Read the model definition and answer for the solid it produces. Units are mm, in the model's axes. Face numbers are marked on the shaded views. A direction names the side the tool comes from. Coordinates: 2 decimals unless noted, no trailing zeros. Order: outer loops, then holes, each group sorted by start corner. A loop starts at its lowest first (then second) coordinate and runs counter-clockwise, first axis right, second up. Notation, with made-up numbers: (77.25, -15) -> (81.25, -15) arc R23 cw to (81.25, 8) -> close; hole circle Ø9 at (78.25, -37). An arc over 180 degrees is marked (long way). Use CSV: the item, a comma, the result in double quotes.
Autodesk Inventor part; units mm, degrees
ref_plane "YZ Plane" through (0, 0, 0) normal (1, 0, 0) x (0, 1, 0)
ref_plane "XZ Plane" through (0, 0, 0) normal (0, 1, 0) x (-1, 0, 0)
ref_plane "XY Plane" through (0, 0, 0) normal (0, 0, 1) x (1, 0, 0)
sketch "Sketch1" plane through (0, 0, 0) normal (0, 0, 1) x (1, 0, 0)
  circle A0 centre (0, 0) radius 16 construction
  line L0 (17.5, 17.5) -> (-17.5, -17.5) construction
  line L1 (-17.5, 17.5) -> (17.5, -17.5) construction
  line L2 (-17, -6) -> (-16.5, -6)
  line L3 (-16, -5.5) -> (-16, 5.5)
  line L4 (-16.5, 6) -> (-17, 6)
  line L5 (-17.5, 12.5) -> (-17.5, 6.5)
  line L6 (-17.5, -6.5) -> (-17.5, -12.5)
  arc A1 (-16.5, -6) -> (-16, -5.5) centre (-16.5, -5.5) ccw
  arc A2 (-16, 5.5) -> (-16.5, 6) centre (-16.5, 5.5) ccw
  arc A3 (-17.5, 6.5) -> (-17, 6) centre (-17, 6.5) ccw
  arc A4 (-17, -6) -> (-17.5, -6.5) centre (-17, -6.5) ccw
  line L7 (6, -17) -> (6, -16.5)
  line L8 (5.5, -16) -> (-5.5, -16)
  line L9 (-6, -16.5) -> (-6, -17)
  arc A5 (6, -16.5) -> (5.5, -16) centre (5.5, -16.5) ccw
  arc A6 (-5.5, -16) -> (-6, -16.5) centre (-5.5, -16.5) ccw
  arc A7 (-6.5, -17.5) -> (-6, -17) centre (-6.5, -17) ccw
  arc A8 (6, -17) -> (6.5, -17.5) centre (6.5, -17) ccw
  line L10 (17, 6) -> (16.5, 6)
  line L11 (16, 5.5) -> (16, -5.5)
  line L12 (16.5, -6) -> (17, -6)
  arc A9 (16.5, 6) -> (16, 5.5) centre (16.5, 5.5) ccw
  arc A10 (16, -5.5) -> (16.5, -6) centre (16.5, -5.5) ccw
  arc A11 (17.5, -6.5) -> (17, -6) centre (17, -6.5) ccw
  arc A12 (17, 6) -> (17.5, 6.5) centre (17, 6.5) ccw
  line L13 (-6, 17) -> (-6, 16.5)
  line L14 (-5.5, 16) -> (5.5, 16)
  line L15 (6, 16.5) -> (6, 17)
  arc A13 (-6, 16.5) -> (-5.5, 16) centre (-5.5, 16.5) ccw
  arc A14 (5.5, 16) -> (6, 16.5) centre (5.5, 16.5) ccw
  arc A15 (6.5, 17.5) -> (6, 17) centre (6.5, 17) ccw
  arc A16 (-6, 17) -> (-6.5, 17.5) centre (-6.5, 17) ccw
  line L16 (12.5, 17.5) -> (6.5, 17.5)
  line L17 (-6.5, 17.5) -> (-12.5, 17.5)
  line L18 (17.5, -12.5) -> (17.5, -6.5)
  line L19 (17.5, 6.5) -> (17.5, 12.5)
  line L20 (-12.5, -17.5) -> (-6.5, -17.5)
  line L21 (6.5, -17.5) -> (12.5, -17.5)
  arc A17 (-17.5, -12.5) -> (-12.5, -17.5) centre (-12.5, -12.5) ccw
  arc A18 (-12.5, 17.5) -> (-17.5, 12.5) centre (-12.5, 12.5) ccw
  arc A19 (17.5, 12.5) -> (12.5, 17.5) centre (12.5, 12.5) ccw
  arc A20 (12.5, -17.5) -> (17.5, -12.5) centre (12.5, -12.5) ccw
  circle A21 centre (0, 0) radius 1.4
  point P0 (16, 0)
  point P1 (0, 0)
  point P2 (-16, 6)
  point P3 (-16, -6)
  point P4 (-16, 0)
  point P5 (-6, -16)
  point P6 (6, -16)
  point P7 (0, -16)
  point P8 (16, -6)
  point P9 (16, 6)
  point P10 (6, 16)
  point P11 (-6, 16)
  point P12 (0, 16)
  dimension "d17" = 16
  dimension "d39" = 35
  dimension "d44" = 12
  dimension "d45" = 0.5
  dimension "d48" = 360
  dimension "d50" = 5
  dimension "d53" = 2.8
extrude "Extrusion6" add sketch "Sketch1" along normal blind 3
properties part number "290814 Forward Outer Endcap" material "Polycarbonate, Clear"
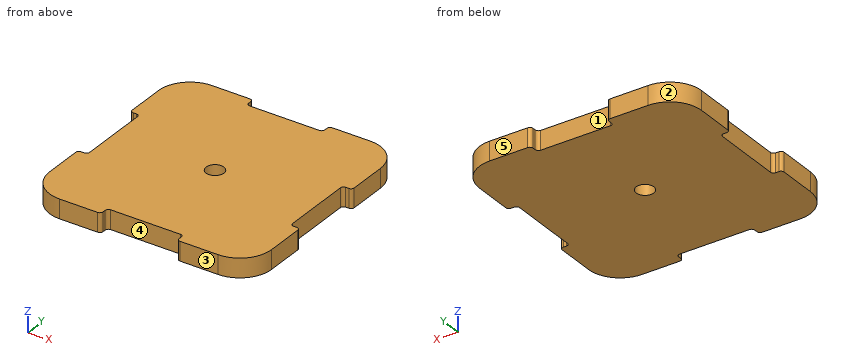
Item 1: A tool of negligible diameter and unlimited length cuts with its end or side. For the marked faces 4 and 5, from which of +Z, -Z, +X, -X, +Y, -Y can it reach the whole face along a straight path? Write none if from no direction.
Return value:
face 4,"+Z, -Z, -Y"
face 5,"+Z, -Z, +X, -X, +Y"
Item 2: The mould has two halves that part along X. Classify the marked faces 1, 2 and 3: +X half, -X half, draft (parallel to the pull), parting line (faces both ways), or undercut.
Return value:
face 1,"undercut"
face 2,"-X half"
face 3,"draft"
Item 3: Find section C-C, the plane y = 3.5. Give the vertices of the cut face in (x, z), then the cut area to 3 significant figures.
Return value:
outline,"(-16, 0) -> (16, 0) -> (16, 3) -> (-16, 3) -> close"
area,"96.0 mm^2"
Item 4: Straight lines are drawn through the part: line 1 along Y through (x, z) = (0, 0.9); line 2 along X through (y, z) = (5, 2.5). For each, find the intervals that lie inside material, in ascending order.
Return value:
line 1,"y = -16 to -1.4, 1.4 to 16"
line 2,"x = -16 to 16"
Item 5: Find section D-D, the plane x = 15. Give the vertices of the cut face in (y, z), then the cut area to 3 significant figures.
Return value:
outline,"(-16.83, 0) -> (16.83, 0) -> (16.83, 3) -> (-16.83, 3) -> close"
area,"101 mm^2"
Item 6: Each of these flat-tipped pins is pushed along its axis until it touches: P1, Ø0.6, axis at y = -17, z = 2, coming from the +X side; P2, Ø1, axis at y = -3.5, z = 1.5, coming from the -X side; P3, Ø1.5, axis at y = -1.5, z = 1.5, coming from the +X side. Where does it stop, or does it pass through?
Return value:
P1,"stops at x = 15.21"
P2,"stops at x = -16"
P3,"stops at x = 16"
Item 7: Find section A-A, the plane x = 0. Give the vertices of the cut face in (y, z), then the cut area to 3 significant figures.
Return value:
outline,"(-16, 0) -> (-1.4, 0) -> (-1.4, 3) -> (-16, 3) -> close; (1.4, 0) -> (16, 0) -> (16, 3) -> (1.4, 3) -> close"
area,"87.6 mm^2"
